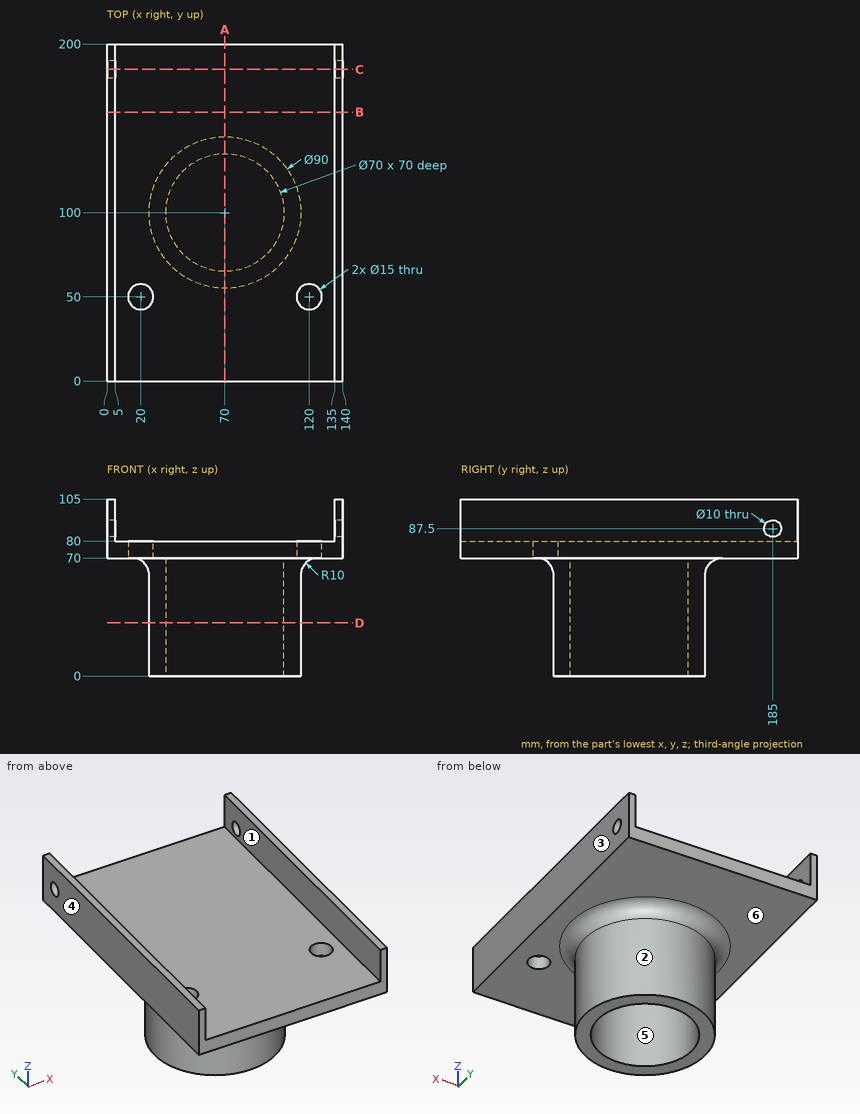
The figure shows three views and two pictorial views of one solid part (mm, origin at its lowest corner). Answer the questions. A direction names the side the tool comes from. Round coordinates to 2 decimals unless told otherwise and drop trailing zeros. Write each loop counter-clockwise with the first axis right and the second up, starting at its lowest first coordinate (ties: lowest second). Pieces come first, ordered by that corner, then holes. Notation, with made-up numbers: M 80.5,-10.5 L 131.5,-10.5 A23 ccw 131.5,11.5 Z; hole C 59.25,-17.5 d11. An arc over 180 degrees is marked long. Write each question's results on one line, items separated by ' | '. Start each with the question number.
(1) The part is cut by section D-D, the plane z = 31.5. Write down the section's boundary in (x, y), and give its area (3 significant figures).
(2) The part is cut by section A-A, the plane x = 70. Write down the section's boundary in (y, z).
(3) The part is cut by section B-B, the plane y = 159.5. Write down the section's boundary in (x, z).
(4) For the marked faces 1 and 2, determine the directions among +Z, -Z, +X, -X, +Y, -Y from which every point of the face is accessible in a straight line to the end or side of a thin tool.
(5) Find the intervals of material crossed by line 1 (Z direction, x = 137.75, y = 185); line 2 (X direction, y = 190, z = 96); line 3 (Y direction, x = 20, z = 72), in increasing order.
(6) The part is cut by section C-C, the plane y = 185. Write down the section's boundary in (x, z), and give its area (3 significant figures).
(7) Each of these flat-tipped pins is pushed along its axis until it touches: P1, Ø12, axis at y = 156, z = 45, coming from the +X side; P2, Ø10, axis at x = 23.5, y = 179, coming from the -Z side; P3, Ø1, axis at x = 74, z = 45, coming from the -Y side; P4, Ø19.5, axis at x = 20, y = 50, coming from the +Z side. Where does it stop, or does it pass through?
(8) Determine the mould class of the marked faces 3, 4, 5 and 6 for opening direction X: +X half, -X half, draft (parallel to the pull), parting line (faces both ways), or undercut.
Worked answers:
1) outline: C 70,100 d90; hole C 70,100 d70 | area: 2,510 mm²
2) outline: M 0,70 L 45,70 A10 cw 55,60 L 55,0 L 65,0 L 65,70 L 135,70 L 135,0 L 145,0 L 145,60 A10 cw 155,70 L 200,70 L 200,80 L 0,80 Z
3) outline: M 0,70 L 140,70 L 140,105 L 135,105 L 135,80 L 5,80 L 5,105 L 0,105 Z
4) face 1: +Z, +Y, -Y | face 2: -Z
5) line 1: z = 70 to 82.5, 92.5 to 105 | line 2: x = 0 to 5, 135 to 140 | line 3: y = 0 to 42.5, 57.5 to 200
6) outline: M 0,70 L 140,70 L 140,82.5 L 135,82.5 L 135,80 L 5,80 L 5,82.5 L 0,82.5 Z; M 0,92.5 L 5,92.5 L 5,105 L 0,105 Z; M 135,92.5 L 140,92.5 L 140,105 L 135,105 Z | area: 1,550 mm²
7) P1: passes through | P2: stops at z = 70 | P3: stops at y = 55.14 | P4: stops at z = 80
8) face 3: +X half | face 4: -X half | face 5: undercut | face 6: draft
